from build123d import *

# Parameters (mm, degrees)
ESBO_O1_R                = 1.5
ESBO_O1_R_2              = 0.75
RESSALTO_EXTRUS_O1_DEPTH = 3


with BuildPart() as part:
    # Esboço1 → Ressalto-extrusão1 (new body)
    with BuildSketch(Plane(origin=(0, 0, 0), x_dir=(1, 0, 0), z_dir=(0, 1, 0))):
        with BuildLine():
            Line((9.52753895, 11.585594571), (9.52753895, 10.546827297))
            Line((9.52753895, 10.546827297), (10.666041157, 10.546827297))
            ThreePointArc((10.666041157, 10.546827297), (-10.110139897, -11.080842534), (9.52753895, 11.585594571))
        make_face()
        with Locations(Location((0, 0, 0), (0, 0, 270))):
            Circle(ESBO_O1_R, mode=Mode.SUBTRACT)
        with Locations(Location((8.625869215, 9.449196698, 0), (0, 0, 270))):
            Circle(ESBO_O1_R_2, mode=Mode.SUBTRACT)
    extrude(amount=RESSALTO_EXTRUS_O1_DEPTH)


solid = part.part
Design review of the part built by this model. Coordinates are the model's own, in mm. Give positions to 0.01 mm unless a question says otherwise; leave off trailing zeros. Loops run counter-clockwise (first coordinate to the right, second up) from the corner with the lowest first, then second, coordinate; pieces in that order, holes last. Notation, with made-up numbers: (23.25, -30) - (79.25, -30) arc R24 ccw to (79.25, 1) - close; hole circle Ø3 at (82.5, 28.25). An arc over 180 degrees is marked (long way). Write item = value, one per line.
1) To check wall thickness, follow line 1 (X direction, y = 1.2, z = 0); line 2 (X direction, y = 0.6, z = -11); line 3 (Z direction, x = 8.5, y = 1.05). State the ranges of each line that lie inside material, in increasing order.
Result sheet:
line_1 = -15 to -1.5, 1.5 to 15
line_2 = -10.2 to 9.53
line_3 = -12.36 to -10.19, -8.71 to 12.36
2) Draft analysis for pull direction X (two halves, no side actions). For faces 1 (the face through (8.17, 1.479, -10.044)), 2 (the face through (10, 1, -10.547)), 3 (the face through (9.528, 1, -11)), 4 (the face through (0.45, 1.48, 1.43)), state which applies: +X half, -X half, draft (parallel to the pull), parting line (faces both ways), or undercut.
Result sheet:
face_1 = undercut
face_2 = draft
face_3 = +X half
face_4 = undercut
3) Take a section at C-C on y = 2.5. State the section outline as (x, z) points, and give its area (3 significant figures).
Result sheet:
outline = (9.53, -11.59) - (9.53, -10.55) - (10.67, -10.55) arc R15 ccw (long way) to start; hole circle Ø3 at (0, 0); hole circle Ø1.5 at (8.63, -9.45)
area = 697 mm2
4) Take a section at D-D on x = -10. State the section outline as (y, z) points, and give its area (3 significant figures).
Result sheet:
outline = (0, -11.18) - (3, -11.18) - (3, 11.18) - (0, 11.18) - close
area = 67.1 mm2
5) Take a section at A-A on z = 0. State the section outline as (x, y) points, and give its area (3 significant figures).
Result sheet:
outline = (-15, 0) - (-1.5, 0) - (-1.5, 3) - (-15, 3) - close; (1.5, 0) - (15, 0) - (15, 3) - (1.5, 3) - close
area = 81.0 mm2
6) Take a section at B-B on x = 0. State the section outline as (y, z) points, and give its area (3 significant figures).
Result sheet:
outline = (0, -15) - (3, -15) - (3, -1.5) - (0, -1.5) - close; (0, 1.5) - (3, 1.5) - (3, 15) - (0, 15) - close
area = 81.0 mm2
7) Clearance check with flat-ended pins moving along their axes: pin 1 Ø5 at (x, z) = (0, 0) entering from -Y; pin 2 Ø0.8 at (y, z) = (1.5, -11) entering from +X; pin 3 Ø0.6 at (x, y) = (10, 2) entering from -Z. State where each tip first meets the part, or that it passes through.
Result sheet:
pin_1 = 0
pin_2 = 9.53
pin_3 = -10.55
